Model file for the job. Use its own axes, mm. Face numbers are marked on the shaded views. A direction names the side the tool comes from. Coordinates: 2 decimals unless noted, no trailing zeros. Order: outer loops, then holes, each group sorted by start corner. A loop starts at its lowest first (then second) coordinate and runs counter-clockwise, first axis right, second up.
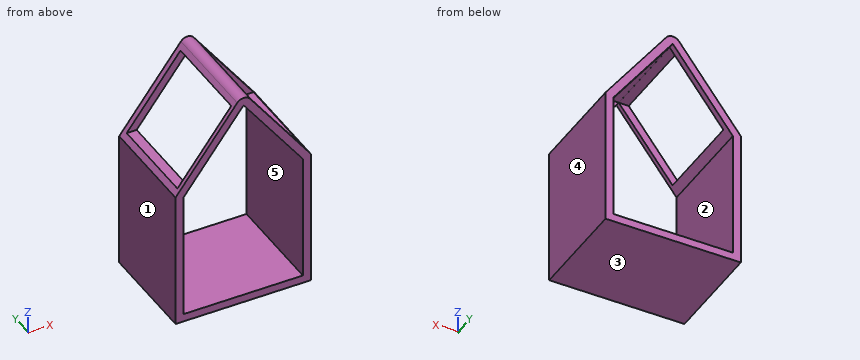
from build123d import *

# Parameters (mm, degrees)
F1_DEPTH      = 165.1
F2_R          = 12.7
F3_W          = 148.7911092117
F3_H          = 113.6830970645
F4_DEPTH      = 168.43995
F4_DEPTH_BACK = 150.70774


with BuildPart() as f1:
    # F0 (on Front) → F1 (new body)
    with BuildSketch(Plane.XZ):
        Polygon((107.244443667, 67.909792846), (0.0752603531, 211.8683984813), (-108.655556333, 67.959965798), (-108.655556333, -152.1984019804), (107.244443667, -152.1984019804), align=None)
        Polygon((94.544443667, -139.4984019804), (-95.955556333, -139.4984019804), (-95.955556333, 63.7015980196), (0, 190.7015980196), (94.544443667, 63.7015980196), align=None, mode=Mode.SUBTRACT)
    extrude(amount=F1_DEPTH)

    # F2
    f2_edges = [f1.edges().sort_by_distance(p)[0] for p in [
        (0.07526, -82.55, 211.868398),
    ]]
    fillet(f2_edges, radius=F2_R)

    # F3 (on Right) → F4 (cut, two sides)
    with BuildSketch(Plane.YZ) as f4_sk:
        with Locations((-83.8478184305, 133.8204629719)):
            Rectangle(F3_W, F3_H)
    extrude(amount=-F4_DEPTH, mode=Mode.SUBTRACT)
    extrude(f4_sk.sketch, amount=F4_DEPTH_BACK, mode=Mode.SUBTRACT)


solid = f1.part
Q1. Cut at B-B, the plane y = -60. List the corners of the cut face in (x, z), plus the area to 3 significant figures.
Established:
outline: (-108.66, -152.2) - (107.24, -152.2) - (107.24, 67.91) - (100.49, 76.98) - (84.66, 76.98) - (94.54, 63.7) - (94.54, -139.5) - (-95.96, -139.5) - (-95.96, 63.7) - (-85.92, 76.98) - (-101.84, 76.98) - (-108.66, 67.96) - close; (-15.95, 190.66) - (-0.03, 190.66) - (0, 190.7) - (0.03, 190.66) - (15.86, 190.66) - (10.19, 198.29) arc R12.7 ccw to (-10.13, 198.36) - close
area: 8,580 mm2
Q2. Which spindle directions (+Z, -Z, +X, -X, +Y, -Y) get a long thin tool onto all of the face, cutting with end or side? Do the marked faces 4 and 5. Say none if no direction does.
Established:
face 4: +Z, -Z, +X, +Y, -Y
face 5: +Y, -Y
Q3. Cut at A-A, the plane z = -57. List the corners of the cut face in (x, y).
Established:
outline: (-108.66, -165.1) - (-95.96, -165.1) - (-95.96, 0) - (-108.66, 0) - close; (94.54, -165.1) - (107.24, -165.1) - (107.24, 0) - (94.54, 0) - close
Q4. Cut at C-C, the plane x = -45. List the corners of the cut face in (y, z), plus the area to 3 significant figures.
Established:
outline: (-165.1, -152.2) - (0, -152.2) - (0, -139.5) - (-165.1, -139.5) - close; (-165.1, 131.14) - (-158.24, 131.14) - (-158.24, 152.21) - (-165.1, 152.21) - close; (-9.45, 131.14) - (0, 131.14) - (0, 152.21) - (-9.45, 152.21) - close
area: 2,440 mm2
Q5. Drop flat-ended pins along their axis: P1, Ø10, axis at y = -146, z = 86.5, coming from the -X side; P2, Ø8, axis at x = 95, y = -112, coming from the +Z side. Give the stop position or say it passes through.
Established:
P1: passes through
P2: stops at z = 76.98
Q6. Probe line 1 (X direction, y = -48, z = -15.5); line 2 (Y direction, x = 92.5, z = 84.5); line 3 (Z direction, x = -96, y = -30). List the from-to ranges inside material, lowest first.
Established:
line 1: x = -108.66 to -95.96, 94.54 to 107.24
line 2: y = -165.1 to -158.24, -9.45 to 0
line 3: z = -152.2 to 76.98
Q7. Cut at D-D, the plane z = 158. List the corners of the cut face in (x, y), plus the area to 3 significant figures.
Established:
outline: (-40.63, -165.1) - (-24.71, -165.1) - (-24.71, -158.24) - (-40.63, -158.24) - close; (-40.63, -9.45) - (-24.71, -9.45) - (-24.71, 0) - (-40.63, 0) - close; (24.34, -165.1) - (40.18, -165.1) - (40.18, -158.24) - (24.34, -158.24) - close; (24.34, -9.45) - (40.18, -9.45) - (40.18, 0) - (24.34, 0) - close
area: 518 mm2
Q8. Mould opens along X. For the marked faces 1, 2 and 3 say: pulls with the +X half, pulls with the -X half, needs draft (parallel to the pull), parting line crosses it, or undercut.
Established:
face 1: pulls with the -X half
face 2: undercut
face 3: needs draft
